Geometry check sheet. Reference: the model listing, model coordinates, mm. Round coordinates to 2 decimals unless told otherwise and drop trailing zeros. Loops run counter-clockwise (first coordinate to the right, second up) from the corner with the lowest first, then second, coordinate; pieces in that order, holes last. Notation, with made-up numbers: M -20,-34 L 3,-34 A27 cw 3,-14 Z; hole C 8.5,51.25 d11. An arc over 180 degrees is marked long. Write item = value, one per line.
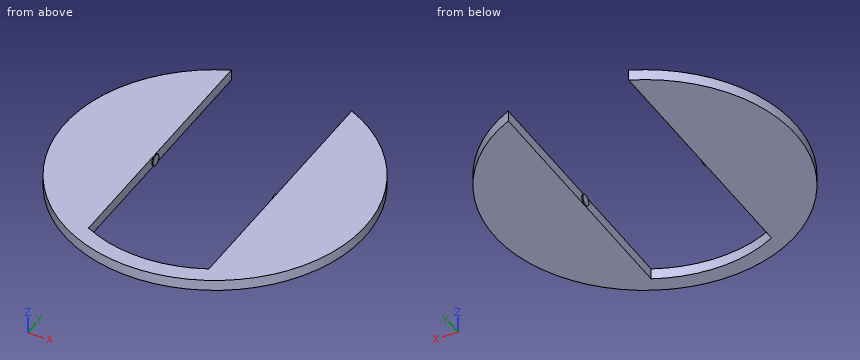
from build123d import *

# Parameters (mm, degrees)
AUFSATZ_LINEAR_AUSTRAGEN1_DEPTH = 20
SKIZZE2_R                       = 10
AUFSATZ_LINEAR_AUSTRAGEN2_DEPTH = 2


with BuildPart() as part:
    # Skizze1 → Aufsatz-Linear austragen1 (new body)
    with BuildSketch(Plane.XY):
        with BuildLine():
            ThreePointArc((-110, 252.041663223), (0, -275), (110, 252.041663223))
            Line((110, 252.041663223), (110, -218.91779279))
            ThreePointArc((110, -218.91779279), (0, -245), (-110, -218.91779279))
            Line((-110, -218.91779279), (-110, 252.041663223))
        make_face()
    extrude(amount=AUFSATZ_LINEAR_AUSTRAGEN1_DEPTH)

    # Skizze2 → Aufsatz-Linear austragen2 (add)
    with BuildSketch(Plane(origin=(-110, 0, 0), x_dir=(0, 0, -1), z_dir=(1, 0, 0))):
        with Locations((-10, 0)):
            Circle(SKIZZE2_R)
    aufsatz_linear_austragen2 = extrude(amount=AUFSATZ_LINEAR_AUSTRAGEN2_DEPTH)

    # Spiegeln1: Aufsatz-Linear austragen2 across plane
    add(aufsatz_linear_austragen2.mirror(Plane(origin=(0, 0, 0), x_dir=(0, 0, 1), z_dir=(1, 0, 0))))


solid = part.part
(1) Depth check by flat-ended pin: pin 1 Ø10 at (y, z) = (-175.5, 5.5) entering from -X; pin 2 Ø10 at (y, z) = (-151.5, 7.5) entering from +X; pin 3 Ø1 at (x, z) = (-98.5, 14.5) entering from +Y. Enter the tip coordinate at first touch or a pass-through.
Result set:
pin_1 = -215.77
pin_2 = 232.73
pin_3 = -224.11
(2) Sectioned sample at D-D on x = 0. Record the cut outline in (y, z), then the cut area to 3 significant figures.
Result set:
outline = M -275,0 L -245,0 L -245,20 L -275,20 Z
area = 600 mm2
(3) Material ranges on line 1 along X through (y, z) = (0, 14.25); line 2 along X through (y, z) = (-145.5, 11.75); line 3 along Y through (x, z) = (111, 10.5), recorded low to high. Write a range as from..to.
Result set:
line_1 = -275..-108, 108..275
line_2 = -233.36..-110, 110..233.36
line_3 = -251.6..251.6
(4) Sectioned sample at A-A on y = 197. Record the cut outline in (x, z).
Result set:
outline = M -191.87,0 L -110,0 L -110,20 L -191.87,20 Z; M 110,0 L 191.87,0 L 191.87,20 L 110,20 Z
(5) Sectioned sample at B-B on z = 10. Record the cut outline in (x, y).
Result set:
outline = M -110,-218.92 L -110,-10 L -108,-10 L -108,10 L -110,10 L -110,252.04 A275 ccw long 110,252.04 L 110,10 L 108,10 L 108,-10 L 110,-10 L 110,-218.92 A245 cw Z
(6) Sectioned sample at C-C on y = -149. Record the cut outline in (x, z), then the cut area to 3 significant figures.
Result set:
outline = M -231.14,0 L -110,0 L -110,20 L -231.14,20 Z; M 110,0 L 231.14,0 L 231.14,20 L 110,20 Z
area = 4,850 mm2
